Model file for the job. Use its own axes, mm. A direction names the side the tool comes from. Coordinates: 2 decimals unless noted, no trailing zeros. Order: outer loops, then holes, each group sorted by start corner. A loop starts at its lowest first (then second) coordinate and runs counter-clockwise, first axis right, second up. Notation, with made-up numbers: (45, 76) -> (102, 76) arc R19 ccw to (102, 100) -> close; hole circle Ø3 at (24.25, -6.75). An arc over 180 degrees is marked (long way). Use CSV: the item, a comma, the result in double quotes. Start each with the question number.
(1) Cut at C-C on x = 8.5. Write the cut outline in (y, z), plus the area to 3 significant figures.
(2) Tool access for faces 5 (the flat face through (0, 28, 2)), 6 (the flat face through (10.5, 11, 0)), 7 (the flat face through (12.5, 14, 2)), 8 (the flat face through (0, 0, 11)), 9 (the flat face through (-18.5, 17, -10)): list every direction of +Z, -Z, +X, -X, +Y, -Y with a clear straight run to the whole face (end or side of a thin tool).
(3) Probe L1, parallel to Y at x = -15.5, z = -9.95; L2, parallel to X at y = 14.5, z = 1; L3, parallel to X at y = 21, z = 11. List the from-to ranges inside material, lowest first.
(4) Pin check, flat tips, straight feed: pin 1 Ø5 at (x, y) = (-15.5, 5) entering from +Z; pin 2 Ø4 at (y, z) = (30.5, -4) entering from +X; pin 3 Ø6.5 at (x, y) = (0.5, 14.5) entering from -Z; pin 4 Ø8 at (y, z) = (11.5, 2.5) entering from +X. Stop position of each tip, or through.
(5) Cut at B-B on x = -15.5. Write the cut outline in (y, z), plus the area to 3 significant figures.
(6) Cut at A-A on y = 5. Write the cut outline in (x, z), plus the area to 3 significant figures.
(7) Cut at D-D on y = 9.5. Write the cut outline in (x, z).
(8) Pull direction X, two halves, no side cores. Call faces 1 (the flat face through (0, 34, -10)), 2 (the flat face through (0, 23, -1)), 3 (the flat face through (-12.5, 14, 2)), 4 (the cylindrical face through (-14, 31, -10)): pulls with the +X half, pulls with the -X half, needs draft (parallel to the pull), parting line crosses it, or undercut.
```python
from build123d import *

# Parameters (mm, degrees)
SKETCH_1_W          = 25
SKETCH_1_H          = 25
EXTRUDE_1_DEPTH     = 25
SHELL_2_T           = -2
SKETCH_2_W          = 21
SKETCH_2_H          = 23
CUT_EXTRUDE_1_DEPTH = 25
SKETCH_3_W          = 25
SKETCH_3_H          = 25
EXTRUDE_2_DEPTH     = 3
EXTRUDE_3_DEPTH     = 4
CUT_EXTRUDE_2_DEPTH = 1
SKETCH_7_R          = 1.5
CUT_EXTRUDE_3_DEPTH = 46.543934832


with BuildPart() as part:
    # 草图1 → 凸台-拉伸1 (new body)
    with BuildSketch(Plane(origin=(0, 0, 0), x_dir=(1, 0, 0), z_dir=(0, 1, 0))):
        Rectangle(SKETCH_1_W, SKETCH_1_H)
    extrude(amount=EXTRUDE_1_DEPTH)

    # 抽壳2
    shell_2_openings = [part.faces().sort_by_distance(p)[0] for p in [
        (0, 12.5, -12.5),
    ]]
    offset(amount=SHELL_2_T, openings=shell_2_openings, kind=Kind.INTERSECTION)

    # 草图2 → 切除-拉伸1 (cut)
    with BuildSketch(Plane(origin=(0, 2, 0), x_dir=(1, 0, 0), z_dir=(0, 1, 0))):
        with Locations((0, 1)):
            Rectangle(SKETCH_2_W, SKETCH_2_H)
    extrude(amount=-CUT_EXTRUDE_1_DEPTH, mode=Mode.SUBTRACT)

    # 草图3 → 凸台-拉伸2 (add)
    with BuildSketch(Plane(origin=(0, 25, 0), x_dir=(1, 0, 0), z_dir=(0, 1, 0))):
        Rectangle(SKETCH_3_W, SKETCH_3_H)
    extrude(amount=EXTRUDE_2_DEPTH)

    # 草图5 → 凸台-拉伸3 (add)
    with BuildSketch(Plane(origin=(0, 0, -12.5), x_dir=(-1, 0, 0), z_dir=(0, 0, -1))):
        Polygon((18.5, 0), (18.5, 34), (-18.5, 34), (-18.5, 0), (-12.5, 0), (-12.5, 28), (12.5, 28), (12.5, 0), align=None)
    extrude(amount=-EXTRUDE_3_DEPTH)

    # 草图6 → 切除-拉伸2 (cut)
    with BuildSketch(Plane(origin=(0, 0, -12.5), x_dir=(-1, 0, 0), z_dir=(0, 0, -1))):
        Polygon((10.5, 0), (18.5, 0), (18.5, 34), (-18.5, 34), (-18.5, 0), (-10.5, 0), (-10.5, 23), (10.5, 23), align=None)
    extrude(amount=-CUT_EXTRUDE_2_DEPTH, mode=Mode.SUBTRACT)

    # 草图7 → 切除-拉伸3 (cut, through all)
    with BuildSketch(Plane(origin=(0, 0, -11.5), x_dir=(-1, 0, 0), z_dir=(0, 0, -1))):
        with Locations((-15.5, 5)):
            Circle(SKETCH_7_R)
        with Locations((-15.5, 31)):
            Circle(SKETCH_7_R)
        with Locations((15.5, 5)):
            Circle(SKETCH_7_R)
        with Locations((15.5, 31)):
            Circle(SKETCH_7_R)
    extrude(amount=-CUT_EXTRUDE_3_DEPTH, mode=Mode.SUBTRACT)


solid = part.part
```
Outcome:
1,outline,"(0, 10.5) -> (23, 10.5) -> (23, -11.5) -> (34, -11.5) -> (34, -8.5) -> (28, -8.5) -> (28, 12.5) -> (0, 12.5) -> close"
1,area,"184 mm2"
2,face 5,"+Z, +X, -X, +Y"
2,face 6,"-Z, -Y"
2,face 7,"+Z, +X, +Y, -Y"
2,face 8,"+Z, -Z, +X, -X, -Y"
2,face 9,"+Z, -Z, -X, +Y, -Y"
3,L1,"0 to 3.5, 6.5 to 29.5, 32.5 to 34"
3,L2,"-12.5 to -10.5, 10.5 to 12.5"
3,L3,"-12.5 to 12.5"
4,pin 1,"z = -8.5"
4,pin 2,"through"
4,pin 3,"z = 10.5"
4,pin 4,"x = 12.5"
5,outline,"(0, -11.5) -> (3.5, -11.5) -> (3.5, -8.5) -> (0, -8.5) -> close; (6.5, -11.5) -> (29.5, -11.5) -> (29.5, -8.5) -> (6.5, -8.5) -> close; (32.5, -11.5) -> (34, -11.5) -> (34, -8.5) -> (32.5, -8.5) -> close"
5,area,"84.0 mm2"
6,outline,"(-18.5, -11.5) -> (-17, -11.5) -> (-17, -8.5) -> (-18.5, -8.5) -> close; (-14, -11.5) -> (-10.5, -11.5) -> (-10.5, 10.5) -> (10.5, 10.5) -> (10.5, -11.5) -> (14, -11.5) -> (14, -8.5) -> (12.5, -8.5) -> (12.5, 12.5) -> (-12.5, 12.5) -> (-12.5, -8.5) -> (-14, -8.5) -> close; (17, -11.5) -> (18.5, -11.5) -> (18.5, -8.5) -> (17, -8.5) -> close"
6,area,"156 mm2"
7,outline,"(-18.5, -11.5) -> (-10.5, -11.5) -> (-10.5, 10.5) -> (10.5, 10.5) -> (10.5, -11.5) -> (18.5, -11.5) -> (18.5, -8.5) -> (12.5, -8.5) -> (12.5, 12.5) -> (-12.5, 12.5) -> (-12.5, -8.5) -> (-18.5, -8.5) -> close"
8,face 1,"needs draft"
8,face 2,"undercut"
8,face 3,"pulls with the -X half"
8,face 4,"undercut"
